The listing builds one solid part. Answer for the finished solid, in the listing's coordinates (mm). Coordinates: 2 decimals unless noted, no trailing zeros. Order: outer loops, then holes, each group sorted by start corner. A loop starts at its lowest first (then second) coordinate and runs counter-clockwise, first axis right, second up. Notation, with made-up numbers: M -2.5,-24.5 L 55.5,-24.5 A18 ccw 55.5,-4.5 Z; hole C 40.5,44.5 d1. An arc over 180 degrees is marked long. One line per item, written item: value. Start each with the question number.
Q1. The part is cut by section B-B on x = -43.5. Give the vertices of the cut face in (y, z) (3 decimals), then the cut area to 3 significant figures.
Q2. Each of these flat-tipped pins is pushed along its axis until it touches: pin 1 Ø3 at (x, z) = (-38.1, -9.06) entering from -Y; pin 2 Ø1.6 at (x, y) = (-3, 1) entering from +Z; pin 3 Ø1.6 at (x, y) = (-41.5, 1) entering from -Z. Where does it stop, or does it pass through?
Q3. Straight lines are drawn through the part: line 1 along Z through (x, y) = (-38.1, 2.05) (3 decimals); line 2 along Z through (x, y) = (-48, 1.55); line 3 along Z through (x, y) = (-39.5, 1.7). For each, find the intervals that lie inside material, in ascending order. Write a range as [from, to].
Q4. The part is cut by section A-A on y = 1.3. Give the vertices of the cut face in (x, z) (1 decimal), then the cut area to 3 significant figures.
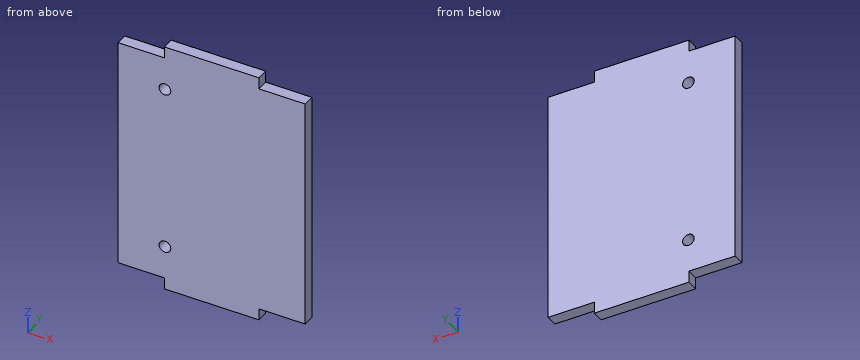
Autodesk Inventor part; units mm, degrees
ref_plane "YZ Plane" through (0, 0, 0) normal (1, 0, 0) x (0, 1, 0)
ref_plane "XZ Plane" through (0, 0, 0) normal (0, 1, 0) x (-1, 0, 0)
ref_plane "XY Plane" through (0, 0, 0) normal (0, 0, 1) x (1, 0, 0)
sketch "Sketch1" plane through (0, 0, 0) normal (0, 1, 0) x (-1, 0, 0)
  line L0 (0, 0) -> (12.5984, 0)
  line L1 (12.5984, 0) -> (12.5984, 3.175)
  line L2 (12.5984, 3.175) -> (38.2016, 3.175)
  line L3 (38.2016, 3.175) -> (38.2016, 0)
  line L4 (38.2016, 0) -> (50.8, 0)
  line L5 (50.8, 0) -> (50.8, -63.5)
  line L6 (50.8, -63.5) -> (38.2016, -63.5)
  line L7 (38.2016, -63.5) -> (38.2016, -66.675)
  line L8 (38.2016, -66.675) -> (12.5984, -66.675)
  line L9 (12.5984, -66.675) -> (12.5984, -63.5)
  line L10 (12.5984, -63.5) -> (0, -63.5)
  line L11 (0, -63.5) -> (0, 0)
  circle A0 centre (38.1, -9.0551) radius 1.5875
  circle A1 centre (38.1, -54.4449) radius 1.5875
  dimension "d0" = 12.5984
  dimension "d1" = 3.175
  dimension "d2" = 25.6032
  dimension "d3" = 63.5
  dimension "d4" = 3.175
  dimension "d5" = 50.8
  dimension "d6" = 3.175
  dimension "d7" = 3.175
  dimension "d8" = 45.3898
  dimension "d9" = 12.7
  dimension "d10" = 9.0551
extrude "Extrusion1" add sketch "Sketch1" along normal blind 3.175
equation "\"d10\" = -0.5 * d8 + 0.5 * d3"
properties part number "top"
Output:
1. outline: M 0,-63.5 L 3.175,-63.5 L 3.175,0 L 0,0 Z
1. area: 202 mm^2
2. pin 1: passes through
2. pin 2: stops at z = 0
2. pin 3: stops at z = -63.5
3. line 1: z = [-66.675, -56.032], [-52.857, -10.643], [-7.468, 3.175]
3. line 2: z = [-63.5, 0]
3. line 3: z = [-63.5, -55.19], [-53.7, -9.8], [-8.31, 0]
4. outline: M -50.8,-63.5 L -38.2,-63.5 L -38.2,-66.7 L -12.6,-66.7 L -12.6,-63.5 L 0,-63.5 L 0,0 L -12.6,0 L -12.6,3.2 L -38.2,3.2 L -38.2,0 L -50.8,0 Z; hole C -38.1,-54.4 d3.2; hole C -38.1,-9.1 d3.2
4. area: 3,370 mm^2
